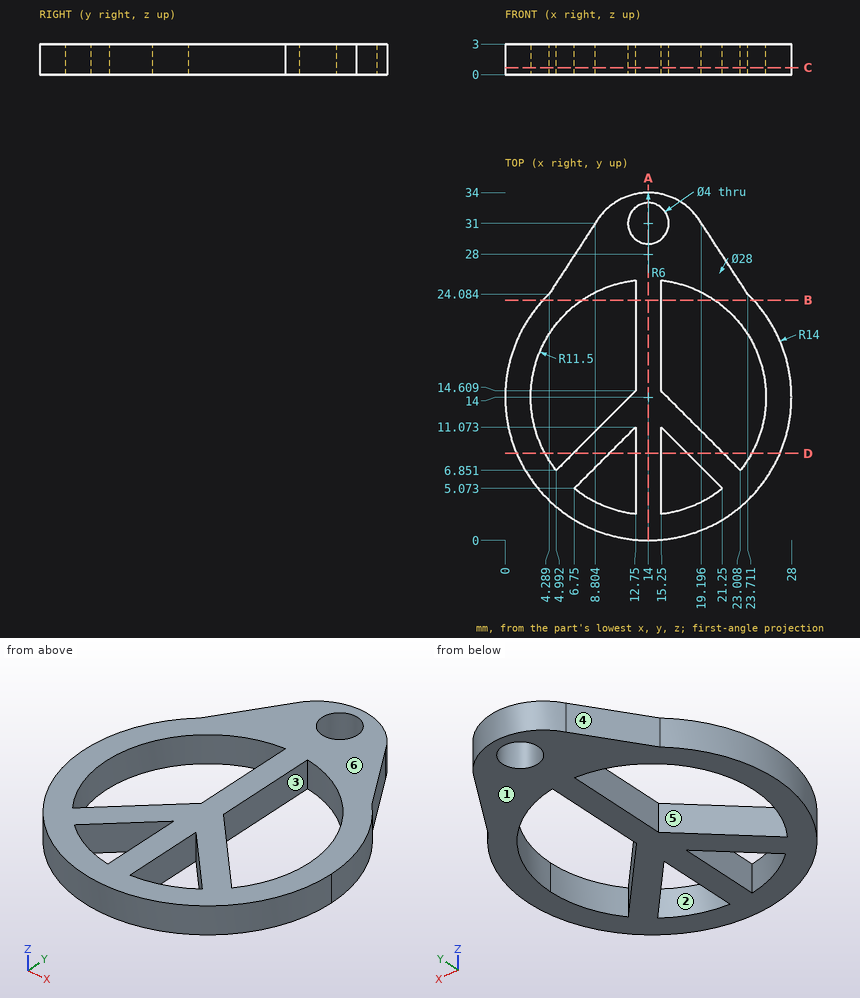
Answer from the drawing. Dimensions are ordinates in mm from the lowest x, y and z of the part. A direction names the side the tool comes from. Give positions to 0.01 mm unless a question says otherwise; leave off trailing zeros. Loops run counter-clockwise (first coordinate to the right, second up) from the corner with the lowest first, then second, coordinate; pieces in that order, holes last.
Item 1: Find the intervals of material crossed by line 1 along X through (y, z) = (31, 0.95) (1 decimal); line 2 along Y through (x, z) = (14, 1.85); line 3 along Y through (x, z) = (17.75, 2.55) (1 decimal), in increasing order.
Item 2: The part is cut by section A-A (x = 14). Write down the section's boundary in (y, z).
Item 3: The part is cut by section B-B (y = 23.5). Write down the section's boundary in (x, z).
Item 4: Each of these flat-tipped pins is pushed along its axis until it touches: pin 1 Ø1.5 at (x, z) = (10, 2) entering from +Y; pin 2 Ø1.5 at (y, z) = (6.5, 2) entering from +X (1 decimal); pin 3 Ø5 at (x, y) = (14, 31) entering from +Z; pin 4 Ø1.5 at (x, z) = (5.5, 2) entering from +Y. Where does it stop, or does it pass through?
Item 5: The mould has two halves that part along Y. Classify the marked faces 1, 2, 3 and 4: released by +Y, released by -Y, zero draft, split by the parting line, or undercut.
Item 6: The part is cut by section D-D (y = 8.5). Give the number of separate pieces and of enclosed holes in the cut face.
Item 7: The part is cut by section C-C (z = 0.7). Write down the section's boundary in (x, y), and give its area (3 significant figures).
Item 8: For the marked faces 5 and 6, determine the directions among +Z, -Z, +X, -X, +Y, -Y from which every point of the face is accessible in a straight line to the end or side of a thin tool.
Taken from the geometry:
1. line 1: x = 8.8 to 12, 16 to 19.2
1. line 2: y = 0 to 29, 33 to 34
1. line 3: y = 0.5 to 3.1, 8.6 to 12.1, 24.9 to 32.7
2. outline: (0, 0) - (29, 0) - (29, 3) - (0, 3) - close; (33, 0) - (34, 0) - (34, 3) - (33, 3) - close
3. outline: (3.72, 0) - (7.52, 0) - (7.52, 3) - (3.72, 3) - close; (12.75, 0) - (15.25, 0) - (15.25, 3) - (12.75, 3) - close; (20.48, 0) - (24.28, 0) - (24.28, 3) - (20.48, 3) - close
4. pin 1: stops at y = 33.04
4. pin 2: stops at x = 26.3
4. pin 3: stops at z = 3
4. pin 4: stops at y = 27.09
5. face 1: zero draft
5. face 2: undercut
5. face 3: undercut
5. face 4: released by +Y
6. separate pieces: 5
6. enclosed holes: 0
7. outline: (4.29, 24.08) arc R14 ccw (long way) to (23.71, 24.08) - (19.2, 31) arc R6 ccw to (8.8, 31) - close; hole (4.99, 6.85) - (12.75, 14.61) - (12.75, 25.43) arc R11.5 ccw to start; hole (6.75, 5.07) arc R11.5 ccw to (12.75, 2.57) - (12.75, 11.07) - close; hole circle Ø4 at (14, 31); hole (15.25, 2.57) arc R11.5 ccw to (21.25, 5.07) - (15.25, 11.07) - close; hole (15.25, 14.61) - (23.01, 6.85) arc R11.5 ccw to (15.25, 25.43) - close
7. area: 367 mm2
8. face 5: +Z, -Z
8. face 6: +Z, +X, -X, +Y, -Y
